Verification items for the finished model (mm, model axes). Face numbers are marked on the shaded views. A direction names the side the tool comes from. Coordinates: 2 decimals unless noted, no trailing zeros. Write each loop counter-clockwise with the first axis right and the second up, starting at its lowest first coordinate (ties: lowest second). Pieces come first, ordered by that corner, then holes. Notation, with made-up numbers: M -34,5 L -13,5 A22 ccw -13,39 Z; hole C 70,-15 d1. An arc over 180 degrees is marked long. Answer in a Markdown table with one row per item.
from build123d import *

# Parameters (mm, degrees)
SKETCH1_W                      = 30
SKETCH1_H                      = 8
BOSS_EXTRUDE1_DEPTH            = 10
CBORE_FOR_M3_SHCS2_D           = 3.2
CBORE_FOR_M3_SHCS2_CBORE_D     = 6.5
CBORE_FOR_M3_SHCS2_CBORE_DEPTH = 3
TAP_DRILL_FOR_M3X0_5_TAP1_D    = 2.5
FILLET1_R                      = 0.5


with BuildPart() as part:
    # Sketch1 → Boss-Extrude1 (new body)
    with BuildSketch(Plane(origin=(0, 0, 0), x_dir=(1, 0, 0), z_dir=(0, 1, 0))):
        Rectangle(SKETCH1_W, SKETCH1_H)
    extrude(amount=BOSS_EXTRUDE1_DEPTH)

    # CBORE for M3 SHCS2 (through all)
    with Locations(Plane(origin=(0, 10, 0), x_dir=(1, 0, 0), z_dir=(0, 1, 0))):
        with Locations((-7.5, 0), (7.5, 0)):
            CounterBoreHole(CBORE_FOR_M3_SHCS2_D / 2, CBORE_FOR_M3_SHCS2_CBORE_D / 2, CBORE_FOR_M3_SHCS2_CBORE_DEPTH)

    # Tap Drill for M3x0.5 Tap1 (through all)
    with Locations(Plane.XY.offset(4)):
        with Locations((-11.5, 5), (11.5, 5)):
            Hole(TAP_DRILL_FOR_M3X0_5_TAP1_D / 2)

    # Fillet1
    fillet1_edges = [part.edges().sort_by_distance(p)[0] for p in [
        (-15, 5, -4),
        (15, 5, -4),
        (15, 5, 4),
        (-15, 5, 4),
    ]]
    fillet(fillet1_edges, radius=FILLET1_R)


solid = part.part
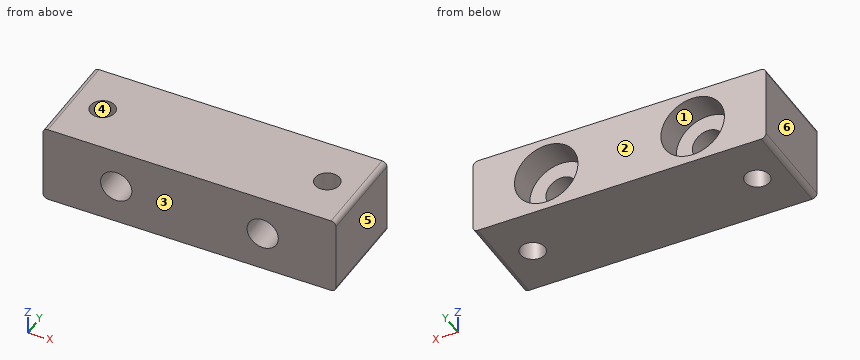
1) Sectioned sample at B-B (x = -11.5). Record the cut outline in (y, z), then the cut area to 3 significant figures.
Response values:
| item | result |
|---|---|
| outline | M 0,-4 L 3.75,-4 L 3.75,4 L 0,4 Z; M 6.25,-4 L 10,-4 L 10,4 L 6.25,4 Z |
| area | 60.0 mm² |
2) Tool access check on the marked faces 1 and 2. Record the directions out of +Z, -Z, +X, -X, +Y, -Y that give a thin tool (end or side, any length) a straight path to the whole face; none if there is none.
Response values:
| item | result |
|---|---|
| face 1 | +Y |
| face 2 | +Z, -Z, +X, -X, +Y |
3) Release check for a two-part mould opening along X. For the marked faces 3, 4, 5 and 6 record: +X half, -X half, draft (parallel to the pull), parting line (faces both ways), or undercut.
Response values:
| item | result |
|---|---|
| face 3 | draft |
| face 4 | undercut |
| face 5 | +X half |
| face 6 | -X half |
4) Sectioned sample at C-C (y = 5). Record the cut outline in (x, z).
Response values:
| item | result |
|---|---|
| outline | M -15,-3.5 A0.5 ccw -14.5,-4 L -12.75,-4 L -12.75,4 L -14.5,4 A0.5 ccw -15,3.5 Z; M -10.25,-4 L 10.25,-4 L 10.25,4 L -10.25,4 Z; M 12.75,-4 L 14.5,-4 A0.5 ccw 15,-3.5 L 15,3.5 A0.5 ccw 14.5,4 L 12.75,4 Z; hole C -7.5,0 d3.2; hole C 7.5,0 d3.2 |
5) Sectioned sample at A-A (z = 0). Record the cut outline in (x, y), then the cut area to 3 significant figures.
Response values:
| item | result |
|---|---|
| outline | M -15,0 L -9.1,0 L -9.1,7 L -10.75,7 L -10.75,10 L -15,10 Z; M -5.9,0 L 5.9,0 L 5.9,7 L 4.25,7 L 4.25,10 L -4.25,10 L -4.25,7 L -5.9,7 Z; M 9.1,0 L 15,0 L 15,10 L 10.75,10 L 10.75,7 L 9.1,7 Z; hole C -11.5,5 d2.5; hole C 11.5,5 d2.5 |
| area | 206 mm² |
6) Thickness scan on L1, parallel to Y at x = 11.5, z = -2.5; L2, parallel to X at y = 4.5, z = -0.25; L3, parallel to X at y = 4.5, z = -3.5. Record the ranges inside material, lowest first. Write a range as [from, to].
Response values:
| item | result |
|---|---|
| L1 | y = [0, 3.75], [6.25, 10] |
| L2 | x = [-15, -12.65], [-10.35, -9.08], [-5.92, 5.92], [9.08, 10.35], [12.65, 15] |
| L3 | x = [-15, -12.65], [-10.35, 10.35], [12.65, 15] |
7) Sectioned sample at D-D (x = -7.5). Record the cut outline in (y, z).
Response values:
| item | result |
|---|---|
| outline | M 0,-4 L 10,-4 L 10,-3.25 L 7,-3.25 L 7,-1.6 L 0,-1.6 Z; M 0,1.6 L 7,1.6 L 7,3.25 L 10,3.25 L 10,4 L 0,4 Z |
8) Depth check by flat-ended pin: pin 1 (2 mm diameter, centred on x = 6, z = 0, fed in from +Y). Enter the tip coordinate at first touch or a pass-through.
Response values:
| item | result |
|---|---|
| pin 1 | stops at y = 7 |
